from build123d import *

# Parameters (mm, degrees)
SKETCH7_W           = 50
SKETCH7_H           = 550
BOSS_EXTRUDE1_DEPTH = 7.5
FILLET1_R           = 18
SKETCH8_R           = 10
CUT_EXTRUDE1_DEPTH  = 324.904692772
SKETCH9_R           = 10
CUT_EXTRUDE2_DEPTH  = 324.904692772


with BuildPart() as part:
    # Sketch7 → Boss-Extrude1 (new, symmetric)
    with BuildSketch(Plane.XY):
        with Locations((12.3, -46.4)):
            Rectangle(SKETCH7_W, SKETCH7_H)
    extrude(amount=BOSS_EXTRUDE1_DEPTH, both=True)

    # Fillet1
    fillet1_edges = [part.edges().sort_by_distance(p)[0] for p in [
        (-12.7, 228.6, 0),
        (37.3, 228.6, 0),
        (37.3, -321.4, 0),
        (-12.7, -321.4, 0),
    ]]
    fillet(fillet1_edges, radius=FILLET1_R)

    # Sketch8 → Cut-Extrude1 (cut, through all)
    with BuildSketch(Plane.XY.offset(7.5)):
        with Locations((12.3, 210.6)):
            Circle(SKETCH8_R)
    extrude(amount=-CUT_EXTRUDE1_DEPTH, mode=Mode.SUBTRACT)

    # Sketch9 → Cut-Extrude2 (cut, through all)
    with BuildSketch(Plane.XY.offset(7.5)):
        with Locations((12.3, -298.842314327)):
            Circle(SKETCH9_R)
    extrude(amount=-CUT_EXTRUDE2_DEPTH, mode=Mode.SUBTRACT)


solid = part.part
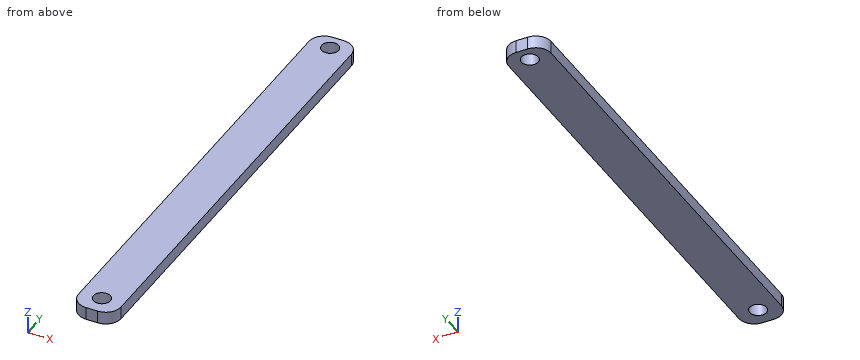
Could you check a few things on this model? Use its own coordinates, in mm. Give positions to 0.01 mm unless a question says otherwise; leave off trailing zeros. Order: outer loops, then holes, each group sorted by start corner. A loop starts at its lowest first (then second) coordinate and runs counter-clockwise, first axis right, second up. Notation, with made-up numbers: M -40,-38.5 L -32,-38.5 A9 cw -32,-26.5 Z; hole C 40.5,30.25 d7. An arc over 180 degrees is marked long. One line per question, with ' | ' between items.
1. I'm going to push flat-ended pins straight in: pin 1 (1.5 mm diameter, centred on x = -2.5, z = -5, fed in from -Y); pin 2 (23 mm diameter, centred on x = 12.3, y = -298.84, fed in from +Z); pin 3 (6 mm diameter, centred on x = 23.5, z = -6, fed in from +Y). Where does each tip first touch, or does it pass through?
Results:
pin 1: y = -319.96 | pin 2: z = 7.5 | pin 3: y = 228.56
2. I want a section at B-B (z = -3.5). List the corners of the cut face in (x, y) for me.
Results:
outline: M -12.7,-303.4 A18 ccw 5.3,-321.4 L 19.3,-321.4 A18 ccw 37.3,-303.4 L 37.3,210.6 A18 ccw 19.3,228.6 L 5.3,228.6 A18 ccw -12.7,210.6 Z; hole C 12.3,-298.84 d20; hole C 12.3,210.6 d20
3. I want a section at A-A (x = 12.3). List the corners of the cut face in (y, z) for me.
Results:
outline: M -321.4,-7.5 L -308.84,-7.5 L -308.84,7.5 L -321.4,7.5 Z; M -288.84,-7.5 L 200.6,-7.5 L 200.6,7.5 L -288.84,7.5 Z; M 220.6,-7.5 L 228.6,-7.5 L 228.6,7.5 L 220.6,7.5 Z
4. I want a section at C-C (x = -7.5). List the corners of the cut face in (y, z) for me, and give its area (3 significant figures).
Results:
outline: M -316.06,-7.5 L 223.26,-7.5 L 223.26,7.5 L -316.06,7.5 Z | area: 8,090 mm²
5. If I drill on line 1 (Y direction, x = 12.3, z = -0.5); line 2 (Y direction, x = 7, z = 5); line 3 (X direction, y = -299, z = -2.75), over which ranges is the centre line in solid material (lowest first)?
Results:
line 1: -321.4 to -308.84, -288.84 to 200.6, 220.6 to 228.6 | line 2: -321.4 to -307.32, -290.36 to 202.12, 219.08 to 228.6 | line 3: -12.7 to 2.3, 22.3 to 37.3
